from build123d import *

# Parameters (mm, degrees)
F0_R            = 10.795
F1_DEPTH        = 6.35
F1_COPIES_COUNT = 3


# Not quite as in the source:
# - a pattern or mirror of a feature is missing from the dataset's text; its kind, count and spacing are read off the source's solid


with BuildPart() as f1:
    # F0 (on Top) → F1 (new body)
    with BuildSketch(Plane.XY):
        with BuildLine():
            Line((-19.05, 63.5), (-19.05, 0))
            ThreePointArc((-19.05, 0), (0, -19.05), (19.05, 0))
            Line((19.05, 0), (19.05, 63.5))
            ThreePointArc((19.05, 63.5), (0, 82.55), (-19.05, 63.5))
        make_face()
        Circle(F0_R, mode=Mode.SUBTRACT)
        with Locations((0, 63.5)):
            Circle(F0_R, mode=Mode.SUBTRACT)
    extrude(amount=F1_DEPTH)

    # F1_copies: F1 ×3 about axis
    f1_copies_axis = Axis((0, 0, 0), (0, 0, 1))


with BuildPart() as f1_1:
    add(f1.part)
    for i in range(1, F1_COPIES_COUNT):
        add(f1.part.rotate(f1_copies_axis, i * 360 / F1_COPIES_COUNT))


solid = f1_1.part
Can you work these out from the model? Positions are in its coordinate system, mm. A direction names the side the tool comes from. Give positions to 0.01 mm unless a question says otherwise; leave off trailing zeros. Order: outer loops, then holes, each group sorted by start corner. A loop starts at its lowest first (then second) coordinate and runs counter-clockwise, first axis right, second up. Notation, with made-up numbers: M 44,-40 L 67,-40 A17 ccw 67,-17 Z; hole C 22.25,6.25 d4. An arc over 180 degrees is marked long. Use a Markdown table: item, result. Add a question column.
Item 1: We'd pull the mould along Y, two halves only. Please class faces 4 (the flat face through (15, -8, 6.35)), 5 (the flat face through (-41.466, -1.943, 3.131)), 6 (the cylindrical face through (44.208, -31.275, 3.131)): +Y half, -Y half, draft (parallel to the pull), parting line (faces both ways), or undercut.
Item 2: Suppose I cut it at C-C (z = 4.5). List the corners of the cut face in (x, y) for me (3 decimals).
Item 3: Suppose I cut it at A-A (y = 0). List the corners of the cut face in (x, z) for me (3 decimals), then the cut area to 3 significant figures.
Item 4: For faces 1 (the flat face through (19.05, 37, 3)), 2 (the flat face through (-19.05, 38, 3)), 3 (the flat face through (-23.052, -35.306, 3.131)), which set-ups out of +Z, -Z, +X, -X, +Y, -Y let a thin tool reach every point of the face, with its end or its side?
Item 5: Suppose I cut it at B-B (x = -62). List the corners of the cut face in (y, z) for me, then the cut area to 3 significant figures.
Item 6: If I drill on L1, parallel to Y at x = 0, z = 4.75 (3 decimals); L2, parallel to X at y = -35.5, z = 2.5; L3, parallel to Y at x = -58, z = 3, over which ranges is the centre line in solid material (lowest first)? Write a range as [from, to].
Item 7: Suppose I cut it at D-D (y = -31.75). List the corners of the cut face in (x, z) for me, then the cut area to 3 significant figures.
Item 8: Will these pins go through, and if not, where does the flat tip stop? pin 1 (3 mm diameter, centred on y = 46, z = 2, fed in from +X); pin 2 (10 mm diameter, centred on x = -4, y = -33, fed in from -Z); pin 3 (1.5 mm diameter, centred on y = 9, z = 1.5, fed in from +X); pin 4 (1 mm diameter, centred on x = -53.5, z = 4, fed in from -Y).
Answer sheet:
| question | item | result |
|---|---|---|
| 1 | face 4 | draft |
| 1 | face 5 | +Y half |
| 1 | face 6 | undercut |
| 2 | outline | M -64.518,-15.252 A19.05 ccw -45.468,-48.248 L 0,-21.997 L 45.468,-48.248 A19.05 ccw 64.518,-15.252 L 19.05,10.999 L 19.05,63.5 A19.05 ccw -19.05,63.5 L -19.05,10.999 Z; hole C -54.993,-31.75 d21.59; hole C 0,0 d21.59; hole C 0,63.5 d21.59; hole C 54.993,-31.75 d21.59 |
| 3 | outline | M -38.1,0 L -10.795,0 L -10.795,6.35 L -38.1,6.35 Z; M 10.795,0 L 38.1,0 L 38.1,6.35 L 10.795,6.35 Z |
| 3 | area | 347 mm² |
| 4 | face 1 | +Z, -Z, +X, +Y |
| 4 | face 2 | +Z, -Z, -X, +Y |
| 4 | face 3 | +Z, -Z, -Y |
| 5 | outline | M -49.46,0 L -39.96,0 L -39.96,6.35 L -49.46,6.35 Z; M -23.54,0 L -13.8,0 L -13.8,6.35 L -23.54,6.35 Z |
| 5 | area | 122 mm² |
| 6 | L1 | y = [-21.997, -10.795], [10.795, 52.705], [74.295, 82.55] |
| 6 | L2 | x = [-73.67, -65.12], [-44.87, -23.39], [23.39, 44.87], [65.12, 73.67] |
| 6 | L3 | y = [-50.56, -42.12], [-21.38, -11.49] |
| 7 | outline | M -74.04,0 L -65.79,0 L -65.79,6.35 L -74.04,6.35 Z; M -44.2,0 L -16.89,0 L -16.89,6.35 L -44.2,6.35 Z; M 16.89,0 L 44.2,0 L 44.2,6.35 L 16.89,6.35 Z; M 65.79,0 L 74.04,0 L 74.04,6.35 L 65.79,6.35 Z |
| 7 | area | 452 mm² |
| 8 | pin 1 | stops at x = 19.05 |
| 8 | pin 2 | passes through |
| 8 | pin 3 | stops at x = 23.81 |
| 8 | pin 4 | stops at y = -50.77 |
